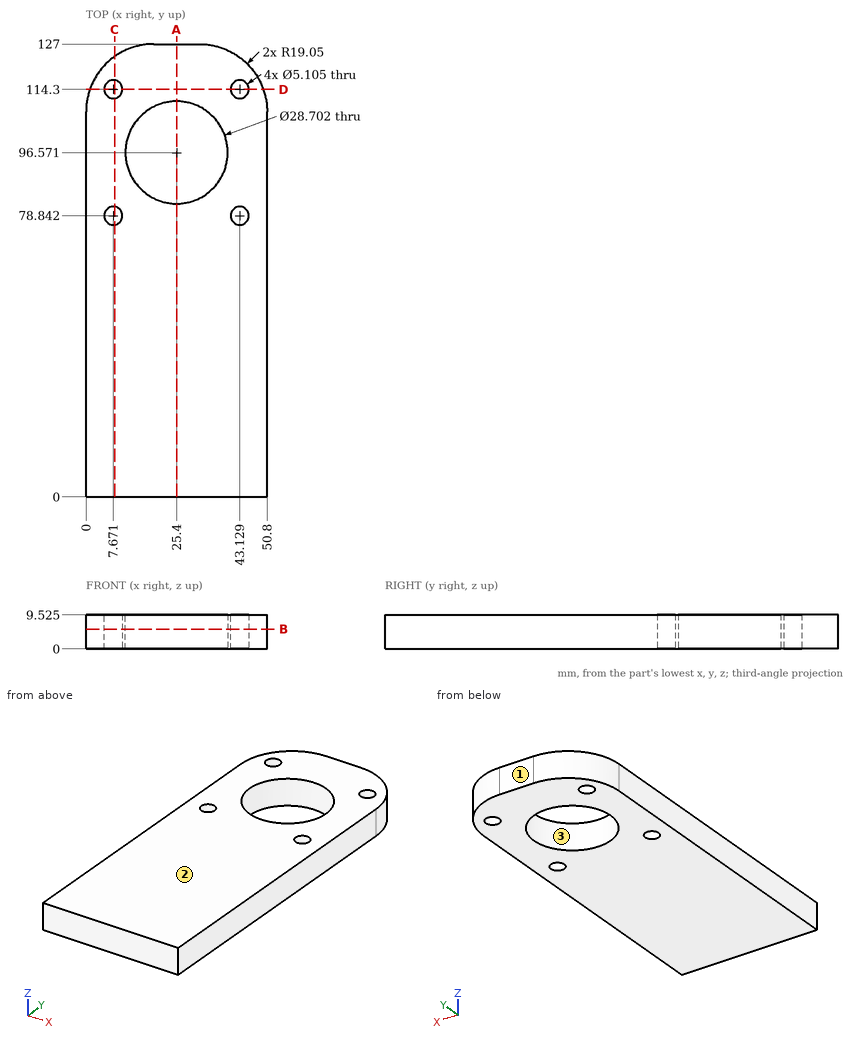
Source: three-view drawing plus pictorial views. Frame: mm from the lowest corner of the part. Coordinates: 2 decimals unless noted, no trailing zeros. Order: outer loops, then holes, each group sorted by start corner. A loop starts at its lowest first (then second) coordinate and runs counter-clockwise, first axis right, second up. Notation, with made-up numbers: M 47,64 L 64,64 A14 cw 64,79 Z; hole C 17,-6.5 d4. An arc over 180 degrees is marked long. Write each question's results on one line, items separated by ' | '. Start each with the question number.
1. Draft query along Y for the marked faces 1, 2 and 3. Return one class per face: +Y half, -Y half, draft (parallel to the pull), parting line (faces both ways), or undercut.
2. Pin query (flat end, axial travel): pin 1 (5 mm diameter, centred on x = 42, z = 4.5, fed in from +Y); pin 2 (3 mm diameter, centred on x = 8, z = 5, fed in from +Y). Return the tip coordinate at first contact, or that it passes through.
3. Section A-A, the plane x = 25.4. Return the cut outline in (y, z) (1 decimal), then the cut area to 3 significant figures.
4. Section B-B, the plane z = 5.5. State how many separate pieces and enclosed holes the cut face has, then the cut area to 3 significant figures.
5. Section D-D, the plane y = 114.3. Return the cut outline in (x, z) (1 decimal).
6. Material intervals for L1, parallel to X at y = 81, z = 3.5 (1 decimal); L2, parallel to Y at x = 10, z = 1.75 (1 decimal); L3, parallel to Y at x = 9, z = 1.5 (1 decimal), sorted ascending.
7. Section C-C, the plane x = 8. Return the cut outline in (y, z) (1 decimal), then the cut area to 3 significant figures.
Solution:
1) face 1: +Y half | face 2: draft | face 3: undercut
2) pin 1: y = 125.35 | pin 2: y = 124.43
3) outline: M 0,0 L 82.2,0 L 82.2,9.5 L 0,9.5 Z; M 110.9,0 L 127,0 L 127,9.5 L 110.9,9.5 Z | area: 936 mm²
4) separate pieces: 1 | enclosed holes: 5 | area: 5,570 mm²
5) outline: M 1.1,0 L 5.1,0 L 5.1,9.5 L 1.1,9.5 Z; M 10.2,0 L 40.6,0 L 40.6,9.5 L 10.2,9.5 Z; M 45.7,0 L 49.7,0 L 49.7,9.5 L 45.7,9.5 Z
6) L1: 0 to 6.3, 9 to 41.8, 44.5 to 50.8 | L2: 0 to 77.8, 79.9 to 113.3, 115.3 to 124.7 | L3: 0 to 76.7, 81 to 112.1, 116.5 to 124.1
7) outline: M 0,0 L 76.3,0 L 76.3,9.5 L 0,9.5 Z; M 81.4,0 L 111.8,0 L 111.8,9.5 L 81.4,9.5 Z; M 116.8,0 L 123.5,0 L 123.5,9.5 L 116.8,9.5 Z | area: 1,080 mm²
